Build history of the part. All positions in model axes, mm. A direction names the side the tool comes from. Give positions to 0.01 mm unless a question says otherwise; leave off trailing zeros. Loops run counter-clockwise (first coordinate to the right, second up) from the corner with the lowest first, then second, coordinate; pieces in that order, holes last. Notation, with made-up numbers: M -8,9.25 L 17,9.25 A24 cw 17,24.25 Z; hole C 3.25,85 d6. An arc over 180 degrees is marked long. Put each result on its own line as item: value.
Autodesk Inventor part; units mm, degrees
ref_plane "YZ Plane" through (0, 0, 0) normal (1, 0, 0) x (0, 1, 0)
ref_plane "XZ Plane" through (0, 0, 0) normal (0, 1, 0) x (-1, 0, 0)
ref_plane "XY Plane" through (0, 0, 0) normal (0, 0, 1) x (1, 0, 0)
sketch "Sketch1" plane through (0, 0, 0) normal (0, 0, 1) x (1, 0, 0)
  circle A0 centre (0, 0) radius 7.5
  dimension "d0" = 15
extrude "Extrusion1" add sketch "Sketch1" along normal blind 55
fillet "Fillet1" radius 7 1 edges at (-7.5, 0, 55)
fillet "Fillet2" radius 7 1 edges at (-7.5, 0, 0)
sketch "Sketch2" plane through (0, 0, 0) normal (1, 0, 0) x (0, 1, 0)
  line L0 (-7.5, 7) -> (-7.5, 48)
  line L1 (-7.5, 37.3739) -> (7.5, 37.3739)
  line L2 (7.5, 37.3739) -> (7.5, 17.3739)
  line L3 (7.5, 17.3739) -> (-7.5, 17.3739)
  line L4 (-7.5, 17.3739) -> (-7.5, 37.3739)
  point P0 (0, 0)
  dimension "d5" = 15
  dimension "d6" = 20
extrude "Extrusion2" add sketch "Sketch2" along normal blind 25.5
sketch "Sketch3" plane through (25.5, 0, 0) normal (1, 0, 0) x (0, 0, -1)
  line L0 (-37.3739, 7.5) -> (-37.3739, -7.5)
  line L1 (-37.3739, 0) -> (-27.3739, 0)
  circle A0 centre (-27.3739, 0) radius 1.75
  point P0 (0, 0)
  dimension "d9" = 10
  dimension "d10" = 3.5
extrude "Extrusion3" add sketch "Sketch3" along normal blind 30
sketch "Sketch4" plane through (25.5, 0, 0) normal (1, 0, 0) x (0, 0, -1)
  circle A0 centre (-27.3739, 0) radius 1.75
  circle A1 centre (-27.3739, 0) radius 4
  point P0 (0, 0)
  dimension "d13" = 8
extrude "Extrusion4" add sketch "Sketch4" along normal blind 20
sketch "Sketch5" plane through (0, -7.5, 17.3739) normal (0, -1, 0) x (1, 0, 0)
  point P0 (0, -17.3739)
properties part number "Mic"
Q1. Slice it at A-A (z = 47). List the corners of the cut face in (x, y).
Here are the results:
outline: C 0,0 d15
Q2. Slice it at B-B (x = 44). List the corners of the cut face in (y, z), and give its area (3 significant figures).
Here are the results:
outline: C 0,27.37 d8
area: 50.3 mm²
Q3. Drop flat-ended pins along their axis: pin 1 Ø2 at (x, y) = (31, 3) entering from +Z; pin 2 Ø1.5 at (y, z) = (4, 11.5) entering from +X; pin 3 Ø6 at (x, y) = (26, -3) entering from +Z. Give the stop position or say it passes through.
Here are the results:
pin 1: z = 30.84
pin 2: x = 6.76
pin 3: z = 37.37
Q4. Slice it at C-C (x = 24.5). List the corners of the cut face in (y, z), and give its area (3 significant figures).
Here are the results:
outline: M -7.5,17.37 L 7.5,17.37 L 7.5,37.37 L -7.5,37.37 Z
area: 300 mm²
Q5. Probe line 1 (Z direction, x = 28, y = -0.25); line 2 (Z direction, x = 13, y = 3.5); line 3 (X direction, y = 1.5, z = 43). List the from-to ranges inside material, lowest first. Write a range as from..to.
Here are the results:
line 1: 23.38..31.37
line 2: 17.37..37.37
line 3: -7.35..7.35
Q6. Tool access for faces 1 (the flat face through (13, 7.5, 28)), 2 (the cylindrical face through (-7.493, -0.33, 27.213)), 3 (the cylindrical face through (35.36, 2.43, 30.55)): list every direction of +Z, -Z, +X, -X, +Y, -Y with a clear straight run to the whole face (end or side of a thin tool).
Here are the results:
face 1: +Z, -Z, +X, -X, +Y
face 2: none
face 3: +X
